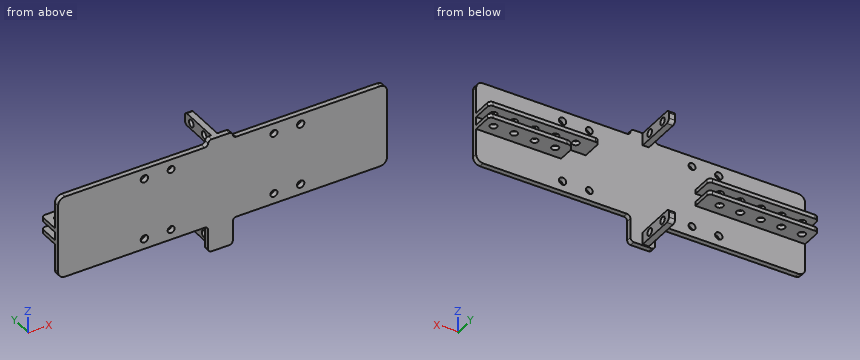
from build123d import *

# Parameters (mm, degrees)
SKETCH_1_W               = 160
SKETCH_1_H               = 40
SKETCH_1_R               = 1.7
EXTRUDE_2_DEPTH          = 2.5
FILLET_2_R               = 3.4
SKETCH_2_W               = 12
SKETCH_2_H               = 16.5
SKETCH_2_H_2             = 6
EXTRUDE_3_DEPTH          = 2.5
FILLET_4_R               = 1.7
FILLET_5_R               = 1.7
SKETCH_3_W               = 3
SKETCH_3_H               = 6
EXTRUDE_4_DEPTH          = 20.5
SKETCH_4_R               = 1.75
CUT_EXTRUDE_1_DEPTH      = 20.5
FILLET_6_R               = 1.7
SKETCH_5_W               = 53.3
SKETCH_5_H               = 2
EXTRUDE_6_DEPTH          = 10.5
CUT_EXTRUDE_2_DEPTH      = 10.5
CUT_EXTRUDE_2_DEPTH_BACK = 10.5
SKETCH_6_R               = 1.75
SKETCH_6_R_2             = 1.7
FILLET_7_R               = 1.7
SKETCH_7_R               = 1.8
CUT_EXTRUDE_3_DEPTH      = 10
SKETCH_8_W               = 10
SKETCH_8_H               = 10.5
SKETCH_8_W_2             = 2
CUT_EXTRUDE_4_DEPTH      = 2
FILLET_8_R               = 3.6


with BuildPart() as part:
    # 草图1 → 凸台-拉伸2 (new body)
    with BuildSketch(Plane(origin=(0, 0, 0), x_dir=(1, 0, 0), z_dir=(0, 1, 0))):
        Rectangle(SKETCH_1_W, SKETCH_1_H)
        with Locations(Location((-25, 15, 0), (0, 0, 270))):
            Circle(SKETCH_1_R, mode=Mode.SUBTRACT)
        with Locations(Location((25, 15, 0), (0, 0, 270))):
            Circle(SKETCH_1_R, mode=Mode.SUBTRACT)
        with Locations(Location((25, -15, 0), (0, 0, 270))):
            Circle(SKETCH_1_R, mode=Mode.SUBTRACT)
        with Locations(Location((-25, -15, 0), (0, 0, 270))):
            Circle(SKETCH_1_R, mode=Mode.SUBTRACT)
    extrude(amount=-EXTRUDE_2_DEPTH)

    # 圆角2
    fillet_2_edges = [part.edges().sort_by_distance(p)[0] for p in [
        (80, -1.25, 20),
        (-80, -1.25, 20),
        (-80, -1.25, -20),
        (80, -1.25, -20),
    ]]
    fillet(fillet_2_edges, radius=FILLET_2_R)

    # 草图2 → 凸台-拉伸3 (add)
    with BuildSketch(Plane(origin=(0, 0, 0), x_dir=(1, 0, 0), z_dir=(0, 1, 0))):
        with Locations((-1, 24.75)):
            Rectangle(SKETCH_2_W, SKETCH_2_H)
        with Locations((-1, -20)):
            Rectangle(SKETCH_2_W, SKETCH_2_H_2)
    extrude(amount=-EXTRUDE_3_DEPTH)

    # 圆角4
    fillet_4_edges = [part.edges().sort_by_distance(p)[0] for p in [
        (-7, -1.25, -33),
        (5, -1.25, -33),
        (-7, -1.25, 23),
        (5, -1.25, 23),
    ]]
    fillet(fillet_4_edges, radius=FILLET_4_R)

    # 圆角5
    fillet_5_edges = [part.edges().sort_by_distance(p)[0] for p in [
        (5, -1.25, 20),
        (-7, -1.25, 20),
        (5, -1.25, -20),
        (-7, -1.25, -20),
    ]]
    fillet(fillet_5_edges, radius=FILLET_5_R)

    # 草图3 → 凸台-拉伸4 (add)
    with BuildSketch(Plane(origin=(0, 0, 0), x_dir=(1, 0, 0), z_dir=(0, 1, 0))):
        with Locations((-2.5, 29.5)):
            Rectangle(SKETCH_3_W, SKETCH_3_H)
        with Locations((-2.5, -20)):
            Rectangle(SKETCH_3_W, SKETCH_3_H)
    extrude(amount=EXTRUDE_4_DEPTH)

    # 草图4 → 切除-拉伸1 (cut)
    with BuildSketch(Plane(origin=(0, 0, 0), x_dir=(0, 0, -1), z_dir=(1, 0, 0))):
        with Locations((-20, 15.5)):
            Circle(SKETCH_4_R)
        with Locations((-20, 5.5)):
            Circle(SKETCH_4_R)
        with Locations((29.5, 15.5)):
            Circle(SKETCH_4_R)
        with Locations((29.5, 5.5)):
            Circle(SKETCH_4_R)
    extrude(amount=-CUT_EXTRUDE_1_DEPTH, mode=Mode.SUBTRACT)

    # 圆角6
    fillet_6_edges = [part.edges().sort_by_distance(p)[0] for p in [
        (-2.5, 20.5, -32.5),
        (-2.5, 20.5, -26.5),
        (-2.5, 20.5, 17),
        (-2.5, 20.5, 23),
    ]]
    fillet(fillet_6_edges, radius=FILLET_6_R)

    # 草图5 → 凸台-拉伸6 (add)
    with BuildSketch(Plane(origin=(0, 0, 0), x_dir=(1, 0, 0), z_dir=(0, 1, 0))):
        with Locations((-53.35, -3)):
            Rectangle(SKETCH_5_W, SKETCH_5_H)
        with Locations((-53.35, 3)):
            Rectangle(SKETCH_5_W, SKETCH_5_H)
        with Locations((53.35, 3)):
            Rectangle(SKETCH_5_W, SKETCH_5_H)
        with Locations((53.35, -3)):
            Rectangle(SKETCH_5_W, SKETCH_5_H)
    extrude(amount=EXTRUDE_6_DEPTH)

    # 草图6 → 切除-拉伸2 (cut, two sides: drawn at the far end of the back side and taken through both)
    with BuildSketch(Plane.XY.offset(-CUT_EXTRUDE_2_DEPTH_BACK)):
        with Locations(Location((-75, 5.5, 0), (0, 0, 180))):
            Circle(SKETCH_6_R)
        with Locations(Location((-65, 5.5, 0), (0, 0, 180))):
            Circle(SKETCH_6_R)
        with Locations(Location((-55, 5.5, 0), (0, 0, 180))):
            Circle(SKETCH_6_R)
        with Locations(Location((-45, 5.5, 0), (0, 0, 180))):
            Circle(SKETCH_6_R)
        with Locations(Location((-35, 5.5, 0), (0, 0, 180))):
            Circle(SKETCH_6_R)
        with Locations(Location((75, 5.5, 0), (0, 0, 180))):
            Circle(SKETCH_6_R_2)
        with Locations(Location((65, 5.5, 0), (0, 0, 180))):
            Circle(SKETCH_6_R_2)
        with Locations(Location((55, 5.5, 0), (0, 0, 180))):
            Circle(SKETCH_6_R_2)
        with Locations(Location((45, 5.5, 0), (0, 0, 180))):
            Circle(SKETCH_6_R_2)
        with Locations(Location((35, 5.5, 0), (0, 0, 180))):
            Circle(SKETCH_6_R_2)
    extrude(amount=CUT_EXTRUDE_2_DEPTH + CUT_EXTRUDE_2_DEPTH_BACK, mode=Mode.SUBTRACT)

    # 圆角7
    fillet_7_edges = [part.edges().sort_by_distance(p)[0] for p in [
        (-80, 10.5, 3),
        (-26.7, 10.5, 3),
        (-80, 10.5, -3),
        (-26.7, 10.5, -3),
        (80, 10.5, -3),
        (26.7, 10.5, -3),
        (80, 10.5, 3),
        (26.7, 10.5, 3),
    ]]
    fillet(fillet_7_edges, radius=FILLET_7_R)

    # 草图7 → 切除-拉伸3 (cut)
    with BuildSketch(Plane(origin=(0, 0, 0), x_dir=(1, 0, 0), z_dir=(0, 1, 0))):
        with Locations(Location((38, 15, 0), (0, 0, 270))):
            Circle(SKETCH_7_R)
        with Locations(Location((38, -15, 0), (0, 0, 270))):
            Circle(SKETCH_7_R)
        with Locations(Location((-38, 15, 0), (0, 0, 270))):
            Circle(SKETCH_7_R)
        with Locations(Location((-38, -15, 0), (0, 0, 270))):
            Circle(SKETCH_7_R)
    extrude(amount=-CUT_EXTRUDE_3_DEPTH, mode=Mode.SUBTRACT)

    # 草图8 → 切除-拉伸4 (cut)
    with BuildSketch(Plane(origin=(0, 0, -4), x_dir=(-1, 0, 0), z_dir=(0, 0, -1))):
        with Locations((-31.7, 5.25)):
            Rectangle(SKETCH_8_W, SKETCH_8_H)
        with Locations((-37.7, 5.25)):
            Rectangle(SKETCH_8_W_2, SKETCH_8_H)
    extrude(amount=-CUT_EXTRUDE_4_DEPTH, mode=Mode.SUBTRACT)

    # 圆角8
    fillet_8_edges = [part.edges().sort_by_distance(p)[0] for p in [
        (38.7, 10.5, -3),
    ]]
    fillet(fillet_8_edges, radius=FILLET_8_R)


solid = part.part
For this review, take the finished solid that the model builds, in its own axes (mm). Coordinates: 2 decimals unless noted, no trailing zeros. Order: outer loops, then holes, each group sorted by start corner. A loop starts at its lowest first (then second) coordinate and runs counter-clockwise, first axis right, second up. Notation, with made-up numbers: (60, 3) - (101, 3) arc R26 cw to (101, 40) - close; hole circle Ø5 at (-10.75, 40.25). An arc over 180 degrees is marked (long way). Answer as CSV lines item,"result". Start each with the question number.
1) Insertion check: P1, Ø4, axis at x = -35, y = 5.5, coming from the -Z side; P2, Ø2, axis at x = 55, y = 5.5, coming from the +Z side; P3, Ø5.5, axis at y = 15.5, z = 20, coming from the +X side; P4, Ø3, axis at x = 29, y = -1, coming from the +Z side. Each pin has a flat end and moves straight along its axis. Give the tip position at first contact, or say it passes through.
2) To check wall thickness, follow line 1 along Y through (x, z) = (45, 3.3); line 2 along Z through (x, y) = (-73, 10); line 3 along Y through (x, z) = (-44.5, -1). State the ranges of each line that lie inside material, in increasing order. Write a range as [from, to].
3) Add section A-A (y = 12). State the section outline as (x, z) points.
4) Add section D-D (x = 75). State the section outline as (y, z) points.
5) Add section B-B (z = 15). State the section outline as (x, y) points.
6) Add section C-C (x = -25). State the section outline as (y, z) points.
Result:
1,P1,"z = -4"
1,P2,"through"
1,P3,"x = -1"
1,P4,"z = 20"
2,line 1,"[-2.5, 3.8], [7.2, 10.5]"
2,line 2,"[-4, -2], [2, 4]"
2,line 3,"[-2.5, 0]"
3,outline,"(-4, -32.5) - (-1, -32.5) - (-1, -26.5) - (-4, -26.5) - close; (-4, 17) - (-1, 17) - (-1, 23) - (-4, 23) - close"
4,outline,"(-2.5, -20) - (0, -20) - (0, -4) - (3.8, -4) - (3.8, -2) - (0, -2) - (0, 2) - (3.8, 2) - (3.8, 4) - (0, 4) - (0, 20) - (-2.5, 20) - close; (7.2, -4) - (10.5, -4) - (10.5, -2) - (7.2, -2) - close; (7.2, 2) - (10.5, 2) - (10.5, 4) - (7.2, 4) - close"
5,outline,"(-80, -2.5) - (-39.8, -2.5) - (-39.8, 0) - (-80, 0) - close; (-36.2, -2.5) - (-26.7, -2.5) - (-26.7, 0) - (-36.2, 0) - close; (-23.3, -2.5) - (23.3, -2.5) - (23.3, 0) - (-23.3, 0) - close; (26.7, -2.5) - (36.2, -2.5) - (36.2, 0) - (26.7, 0) - close; (39.8, -2.5) - (80, -2.5) - (80, 0) - (39.8, 0) - close"
6,outline,"(-2.5, -20) - (0, -20) - (0, -16.7) - (-2.5, -16.7) - close; (-2.5, -13.3) - (0, -13.3) - (0, 13.3) - (-2.5, 13.3) - close; (-2.5, 16.7) - (0, 16.7) - (0, 20) - (-2.5, 20) - close"
